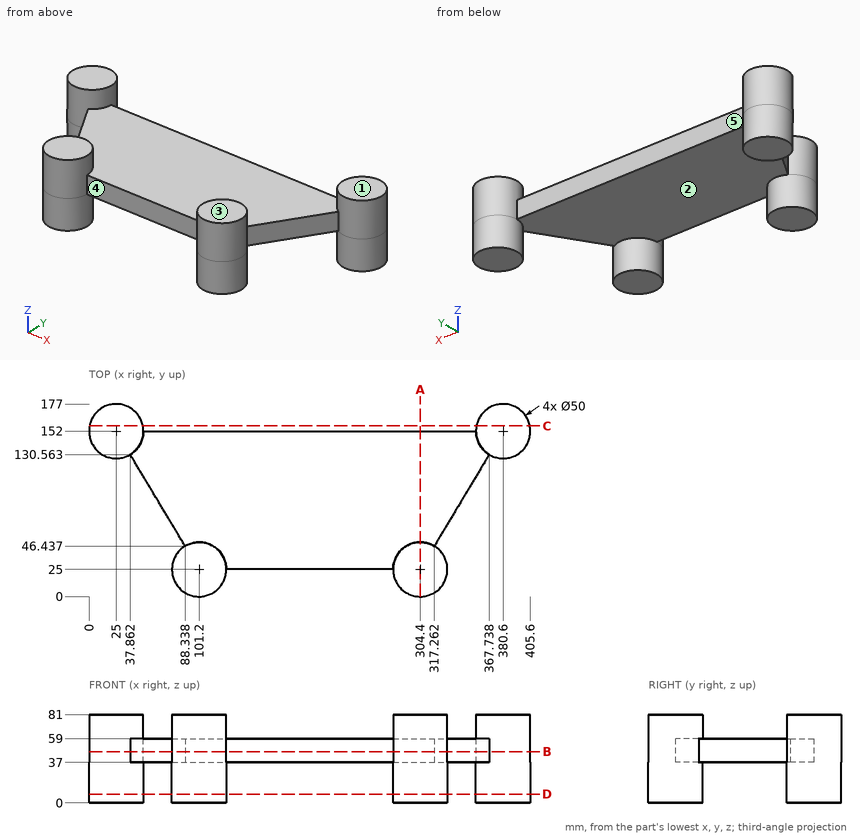
Source: three-view drawing plus pictorial views. Frame: mm from the lowest corner of the part. A direction names the side the tool comes from. Round coordinates to 2 decimals unless told otherwise and drop trailing zeros. Loops run counter-clockwise (first coordinate to the right, second up) from the corner with the lowest first, then second, coordinate; pieces in that order, holes last. Notation, with made-up numbers: M 42.25,35.25 L 89.25,35.25 A38 ccw 89.25,73.25 Z; hole C 40,48 d2. An arc over 180 degrees is marked long. Answer as CSV lines item,"result".
Q1. Contact query for flat-ended pins moving along their axis: pin 1 (1.5 mm diameter, centred on x = 169, y = 141.5, fed in from +Z); pin 2 (3 mm diameter, centred on y = 39, z = 38, fed in from -X); pin 3 (2 mm diameter, centred on x = 176, z = 55.5, fed in from -Y); pin 4 (3 mm diameter, centred on x = 129.5, z = 25.5, fed in from +Y). Output: stop coordinate, or through.
Verdict:
pin 1,"stops at z = 59"
pin 2,"stops at x = 79.55"
pin 3,"stops at y = 25"
pin 4,"passes through"
Q2. Line query: line 1 along Z through (x, y) = (225, 108); line 2 along Y through (x, z) = (251, 49); line 3 along X through (y, z) = (163.5, 12). Output: solid intervals per line, ascending.
Verdict:
line 1,"z = 37 to 59"
line 2,"y = 25 to 152"
line 3,"x = 2.8 to 47.2, 358.4 to 402.8"
Q3. Reachability of the marked faces 3, 4 and 5 from +Z, -Z, +X, -X, +Y, -Y: full face, straight path, thin tool, end or side. Return the list, or none.
Verdict:
face 3,"+Z, +X, -X, +Y, -Y"
face 4,"+Z, -Z, -Y"
face 5,"+Z, -Z, +Y"
Q4. Cut plane D-D (z = 8). Return the cut outline in (x, y), plus the area to 3 significant figures.
Verdict:
outline,"C 25,152 d50; C 101.2,25 d50; C 304.4,25 d50; C 380.6,152 d50"
area,"7,850 mm^2"
Q5. Cut plane B-B (z = 47). Return the cut outline in (x, y), plus the area to 3 significant figures.
Verdict:
outline,"M 37.86,130.56 L 88.34,46.44 A25 ccw long 126.2,25 L 279.4,25 A25 ccw long 317.26,46.44 L 367.74,130.56 A25 ccw long 355.6,152 L 50,152 A25 ccw long Z"
area,"41,400 mm^2"
Q6. Cut plane C-C (y = 157). Return the cut outline in (x, z) (1 decimal), plus the area to 3 significant figures.
Verdict:
outline,"M 0.5,0 L 49.5,0 L 49.5,81 L 0.5,81 Z; M 356.1,0 L 405.1,0 L 405.1,81 L 356.1,81 Z"
area,"7,940 mm^2"
Q7. Pull-direction query (X, two-part tool) for the marked faces 1 and 2; classes: +X half, -X half, draft (parallel to the pull), parting line (faces both ways), or undercut.
Verdict:
face 1,"draft"
face 2,"undercut"
Q8. Cut plane A-A (x = 304.4). Return the cut outline in (y, z), plus the area to 3 significant figures.
Verdict:
outline,"M 0,0 L 50,0 L 50,37 L 152,37 L 152,59 L 50,59 L 50,81 L 0,81 Z"
area,"6,290 mm^2"
